Could you check a few things on this model? Use its own coordinates, in mm. Face numbers are marked on the shaded views. Give positions to 0.01 mm unless a question says otherwise; leave off trailing zeros. Write each loop counter-clockwise with the first axis right and the second up, starting at its lowest first coordinate (ties: lowest second). Pieces come first, ordered by that corner, then holes. Notation, with made-up numbers: M -5,-4 L 43,-4 A21 cw 43,4 Z; hole C 11.5,23.5 d3. An arc over 180 degrees is marked long. One line per item, written item: value.
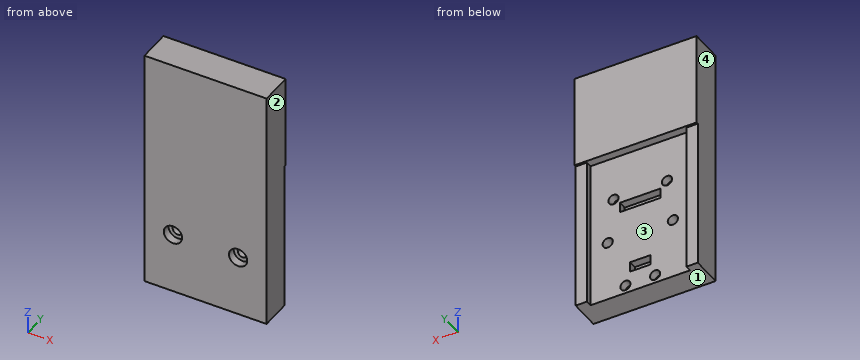
```python
from build123d import *

# Parameters (mm, degrees)
SKETCH1_W           = 30
SKETCH1_H           = 60
SKETCH1_R           = 1.25
BOSS_EXTRUDE1_DEPTH = 6
SKETCH2_R           = 2.25
CUT_EXTRUDE1_DEPTH  = 2
SKETCH3_W           = 2.75
SKETCH3_H           = 60
BOSS_EXTRUDE2_DEPTH = 1.5
SKETCH4_R           = 1.25
SKETCH4_W           = 5
SKETCH4_H           = 2.5
SKETCH4_W_2         = 10
CUT_EXTRUDE2_DEPTH  = 2
SKETCH5_W           = 30
SKETCH5_H           = 23
BOSS_EXTRUDE3_DEPTH = 2


with BuildPart() as part:
    # Sketch1 → Boss-Extrude1 (new body)
    with BuildSketch(Plane(origin=(0, 0, 0), x_dir=(1, 0, 0), z_dir=(0, 1, 0))):
        Rectangle(SKETCH1_W, SKETCH1_H)
        with Locations(Location((-8, 15, 0), (0, 0, 270))):
            Circle(SKETCH1_R, mode=Mode.SUBTRACT)
        with Locations(Location((8, 15, 0), (0, 0, 270))):
            Circle(SKETCH1_R, mode=Mode.SUBTRACT)
    extrude(amount=-BOSS_EXTRUDE1_DEPTH)

    # Sketch2 → Cut-Extrude1 (cut)
    with BuildSketch(Plane(origin=(0, -6, 0), x_dir=(-1, 0, 0), z_dir=(0, -1, 0))):
        with Locations(Location((-8, 15, 0), (0, 0, 90))):
            Circle(SKETCH2_R)
        with Locations(Location((8, 15, 0), (0, 0, 90))):
            Circle(SKETCH2_R)
    extrude(amount=-CUT_EXTRUDE1_DEPTH, mode=Mode.SUBTRACT)

    # Sketch3 → Boss-Extrude2 (add)
    with BuildSketch(Plane(origin=(0, 0, 0), x_dir=(1, 0, 0), z_dir=(0, 1, 0))):
        with Locations((-13.625, 0)):
            Rectangle(SKETCH3_W, SKETCH3_H)
        with Locations((13.625, 0)):
            Rectangle(SKETCH3_W, SKETCH3_H)
    extrude(amount=BOSS_EXTRUDE2_DEPTH)

    # Sketch4 → Cut-Extrude2 (cut)
    with BuildSketch(Plane(origin=(0, 0, 0), x_dir=(1, 0, 0), z_dir=(0, 1, 0))):
        with Locations(Location((-3.65, 28, 0), (0, 0, 270))):
            Circle(SKETCH4_R)
        with Locations(Location((3.65, 28, 0), (0, 0, 270))):
            Circle(SKETCH4_R)
        with Locations(Location((-6.57, 4, 0), (0, 0, 270))):
            Circle(SKETCH4_R)
        with Locations(Location((6.57, 4, 0), (0, 0, 270))):
            Circle(SKETCH4_R)
        with Locations((0, 23.5)):
            Rectangle(SKETCH4_W, SKETCH4_H)
        with Locations((0, 6.71)):
            Rectangle(SKETCH4_W_2, SKETCH4_H)
    extrude(amount=-CUT_EXTRUDE2_DEPTH, mode=Mode.SUBTRACT)

    # Sketch5 → Boss-Extrude3 (add)
    with BuildSketch(Plane(origin=(0, 0, 0), x_dir=(1, 0, 0), z_dir=(0, 1, 0))):
        with Locations((0, -18.5)):
            Rectangle(SKETCH5_W, SKETCH5_H)
    extrude(amount=BOSS_EXTRUDE3_DEPTH)


solid = part.part
```
1) If we section it at C-C, the plane z = 0: Write out the boundary of the cut face in (x, y).
Outcome:
outline: M -15,-6 L 15,-6 L 15,1.5 L 12.25,1.5 L 12.25,0 L -12.25,0 L -12.25,1.5 L -15,1.5 Z
2) I'm going to push flat-ended pins straight in: pin 1 (2 mm diameter, centred on x = 0.5, z = -6.5, fed in from +Y); pin 2 (6 mm diameter, centred on x = -0.5, z = -12.5, fed in from +Y); pin 3 (3 mm diameter, centred on x = 14, z = -15, fed in from +Y). Where does each tip first touch, or does it pass through?
Outcome:
pin 1: stops at y = -2
pin 2: stops at y = 0
pin 3: stops at y = 1.5
3) If we section it at B-B, the plane x = 3.65: Write out the boundary of the cut face in (y, z).
Outcome:
outline: M -6,-30 L 0,-30 L 0,-29.25 L -2,-29.25 L -2,-26.75 L 0,-26.75 L 0,-7.96 L -2,-7.96 L -2,-5.46 L 0,-5.46 L 0,7 L 2,7 L 2,30 L -6,30 Z
4) Please list where these lines run through material, in increasing order: L1, parallel to X at y = -1.4, z = -4; L2, parallel to X at y = -0.35, z = -28; L3, parallel to X at y = 0.25, z = 6.5. Write a range as from..to.
Outcome:
L1: x = -15..-7.82, -5.32..5.32, 7.82..15
L2: x = -15..-4.9, -2.4..2.4, 4.9..15
L3: x = -15..-12.25, 12.25..15
5) If we section it at D-D, the plane z = -24: Write out the boundary of the cut face in (x, y).
Outcome:
outline: M -15,-6 L 15,-6 L 15,1.5 L 12.25,1.5 L 12.25,0 L 2.5,0 L 2.5,-2 L -2.5,-2 L -2.5,0 L -12.25,0 L -12.25,1.5 L -15,1.5 Z
6) We'd pull the mould along X, two halves only. Please class the marked faces 1, 2, 3 and 4: pulls with the +X half, pulls with the -X half, needs draft (parallel to the pull), parting line crosses it, or undercut.
Outcome:
face 1: needs draft
face 2: pulls with the +X half
face 3: undercut
face 4: pulls with the -X half
7) If we section it at A-A, the plane z = -15: Write out the boundary of the cut face in (x, y).
Outcome:
outline: M -15,-6 L -10.25,-6 L -10.25,-4 L -9.25,-4 L -9.25,0 L -12.25,0 L -12.25,1.5 L -15,1.5 Z; M -6.75,-4 L -5.75,-4 L -5.75,-6 L 5.75,-6 L 5.75,-4 L 6.75,-4 L 6.75,0 L -6.75,0 Z; M 9.25,-4 L 10.25,-4 L 10.25,-6 L 15,-6 L 15,1.5 L 12.25,1.5 L 12.25,0 L 9.25,0 Z
